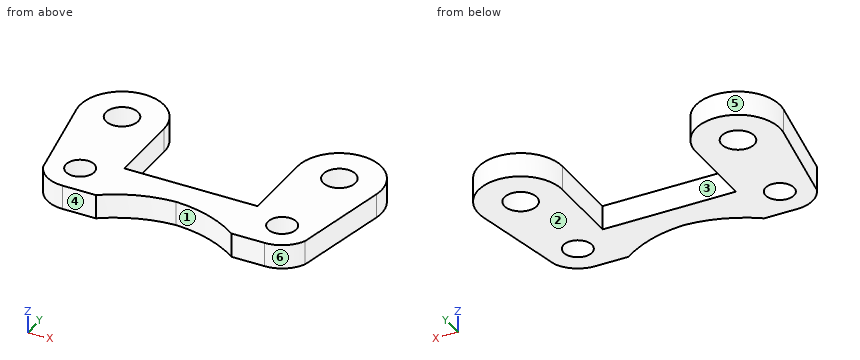
```python
from build123d import *

# Parameters (mm, degrees)
SKETCH1_R           = 4
SKETCH1_R_2         = 3.5
BOSS_EXTRUDE1_DEPTH = 6


with BuildPart() as part:
    # Sketch1 → Boss-Extrude1 (new body)
    with BuildSketch(Plane.XY):
        with BuildLine():
            Line((-25, -41.5), (-16.8, -41.5))
            ThreePointArc((-16.8, -41.5), (-8.828360495, -37.359231669), (0, -35.7))
            ThreePointArc((0, -35.7), (8.828360495, -37.359231669), (16.8, -41.5))
            Line((16.8, -41.5), (25, -41.5))
            ThreePointArc((25, -41.5), (29.432022337, -40.185877375), (32.431413249, -36.668293768))
            Line((32.431413249, -36.668293768), (37.115311752, -12.370570289))
            ThreePointArc((37.115311752, -12.370570289), (27.890603154, -0.04711718), (16.5, -10.401676805))
            Line((16.5, -10.401676805), (16.5, -28.9))
            Line((16.5, -28.9), (-16.5, -28.9))
            Line((-16.5, -28.9), (-16.5, -10.401676805))
            ThreePointArc((-16.5, -10.401676805), (-27.890603154, -0.04711718), (-37.115311752, -12.370570289))
            Line((-37.115311752, -12.370570289), (-32.431413249, -36.668293768))
            ThreePointArc((-32.431413249, -36.668293768), (-29.432022337, -40.185877375), (-25, -41.5))
        make_face()
        with Locations((-26.901676805, -10.401676805)):
            Circle(SKETCH1_R, mode=Mode.SUBTRACT)
        with Locations((-25, -33.369198558)):
            Circle(SKETCH1_R_2, mode=Mode.SUBTRACT)
        with Locations(Location((25, -33.369198558, 0), (0, 0, 180))):
            Circle(SKETCH1_R_2, mode=Mode.SUBTRACT)
        with Locations(Location((26.901676805, -10.401676805, 0), (0, 0, 180))):
            Circle(SKETCH1_R, mode=Mode.SUBTRACT)
    extrude(amount=BOSS_EXTRUDE1_DEPTH)


solid = part.part
```
Input: part model. Units: mm. Frame: model coordinates. Face numbers are marked on the shaded views. A direction names the side the tool comes from. Coordinates: 2 decimals unless noted, no trailing zeros. Loops run counter-clockwise (first coordinate to the right, second up) from the corner with the lowest first, then second, coordinate; pieces in that order, holes last. Notation, with made-up numbers: M 65.25,57 L 89.25,57 A6 cw 89.25,65 Z; hole C 85,89 d6. An arc over 180 degrees is marked long. Answer in a Markdown table with one row per item.
1. Section B-B, the plane z = 3.05. Output: boundary loops of the cut face in (x, y).
Response:
| item | result |
|---|---|
| outline | M -37.12,-12.37 L -32.43,-36.67 A8.13 ccw -25,-41.5 L -16.8,-41.5 A30.74 cw 0,-35.7 A30.74 cw 16.8,-41.5 L 25,-41.5 A8.13 ccw 32.43,-36.67 L 37.12,-12.37 A10.4 ccw long 16.5,-10.4 L 16.5,-28.9 L -16.5,-28.9 L -16.5,-10.4 A10.4 ccw long Z; hole C -26.9,-10.4 d8; hole C -25,-33.37 d7; hole C 25,-33.37 d7; hole C 26.9,-10.4 d8 |
2. Draft query along X for the marked faces 4, 5 and 6. Return one class per face: pulls with the +X half, pulls with the -X half, needs draft (parallel to the pull), parting line crosses it, or undercut.
Response:
| item | result |
|---|---|
| face 4 | needs draft |
| face 5 | undercut |
| face 6 | pulls with the +X half |
3. Section A-A, the plane y = -8. Output: boundary loops of the cut face in (x, z), then the cut area to 3 significant figures.
Response:
| item | result |
|---|---|
| outline | M -37.02,0 L -30.1,0 L -30.1,6 L -37.02,6 Z; M -23.7,0 L -16.78,0 L -16.78,6 L -23.7,6 Z; M 16.78,0 L 23.7,0 L 23.7,6 L 16.78,6 Z; M 30.1,0 L 37.02,0 L 37.02,6 L 30.1,6 Z |
| area | 166 mm2 |
4. Section C-C, the plane y = -25. Output: boundary loops of the cut face in (x, z), then the cut area to 3 significant figures.
Response:
| item | result |
|---|---|
| outline | M -34.68,0 L -16.5,0 L -16.5,6 L -34.68,6 Z; M 16.5,0 L 34.68,0 L 34.68,6 L 16.5,6 Z |
| area | 218 mm2 |
5. Reachability of the marked faces 1, 2 and 3 from +Z, -Z, +X, -X, +Y, -Y: full face, straight path, thin tool, end or side. Return the list, or none.
Response:
| item | result |
|---|---|
| face 1 | +Z, -Z, -Y |
| face 2 | -Z, +X, -X, +Y, -Y |
| face 3 | +Z, -Z, +Y |
6. Section D-D, the plane x = -9.5. Output: boundary loops of the cut face in (y, z), then the cut area to 3 significant figures.
Response:
| item | result |
|---|---|
| outline | M -37.6,0 L -28.9,0 L -28.9,6 L -37.6,6 Z |
| area | 52.2 mm2 |
7. First-contact query: pin 1 (3 mm diameter, centred on y = -23.5, z = 4, fed in from -X); pin 2 (3 mm diameter, centred on x = -17, z = 4, fed in from +Y); pin 3 (3 mm diameter, centred on y = -19, z = 3, fed in from +X); pin 4 (5 mm diameter, centred on x = 26.9, y = -10.4, fed in from -Z). Flat tips, straight axial feed; report the tip coordinate or a pass-through.
Response:
| item | result |
|---|---|
| pin 1 | stops at x = -35.26 |
| pin 2 | stops at y = -4.27 |
| pin 3 | stops at x = 36.13 |
| pin 4 | passes through |
8. Material intervals for line 1 (Y direction, x = -25.5, z = 2.45); line 2 (X direction, y = -14, z = 5.45); line 3 (X direction, y = -33.5, z = 2.2), sorted ascending.
Response:
| item | result |
|---|---|
| line 1 | y = -41.48 to -36.83, -29.91 to -14.15, -6.66 to -0.09 |
| line 2 | x = -36.8 to -28.65, -25.15 to -16.5, 16.5 to 25.15, 28.65 to 36.8 |
| line 3 | x = -33.04 to -28.5, -21.5 to 21.5, 28.5 to 33.04 |
